from build123d import *

# Parameters (mm, degrees)
F0_W        = 9.525
F0_H        = 112.7125
F1_DEPTH    = 1.5875
F2_T1_DEPTH = 26.9875
F4_D        = 3.175


# Not quite as in the source:
# - a fillet or chamfer that OpenCascade refuses, or shapes differently, is made with other operations: its cross-section is extruded or revolved along the edge and cut away or added


with BuildPart() as f1:
    # F0 (on Top) → F1 (new body)
    with BuildSketch(Plane.XY):
        with Locations((0, 56.35625)):
            Rectangle(F0_W, F0_H)
    extrude(amount=F1_DEPTH)

    # F2: fillet of radius 5.08 on 4 edges, made by hand

    # F2_s2 → F2_t1 (cut)
    with BuildSketch(Plane.XY.offset(-12.7)):
        with BuildLine():
            ThreePointArc((-0.3175, 0), (3.2746024484, 1.4878975516), (4.7625, 5.08))
            Line((4.7625, 5.08), (4.7625, 0))
            Line((4.7625, 0), (-0.3175, 0))
        make_face()
        with BuildLine():
            ThreePointArc((-4.7625, 5.08), (-3.2746024484, 1.4878975516), (0.3175, 0))
            Line((0.3175, 0), (-4.7625, 0))
            Line((-4.7625, 0), (-4.7625, 5.08))
        make_face()
        with BuildLine():
            ThreePointArc((-0.3175, 112.7125), (3.2746024484, 111.2246024484), (4.7625, 107.6325))
            Line((4.7625, 107.6325), (4.7625, 112.7125))
            Line((4.7625, 112.7125), (-0.3175, 112.7125))
        make_face()
        with BuildLine():
            ThreePointArc((0.3175, 112.7125), (-3.2746024484, 111.2246024484), (-4.7625, 107.6325))
            Line((-4.7625, 107.6325), (-4.7625, 112.7125))
            Line((-4.7625, 112.7125), (0.3175, 112.7125))
        make_face()
    extrude(amount=F2_T1_DEPTH, mode=Mode.SUBTRACT)

    # F4 (through all)
    with Locations(Plane.XY.offset(1.5875)):
        with Locations((0, 5.08)):
            Hole(F4_D / 2)


solid = f1.part
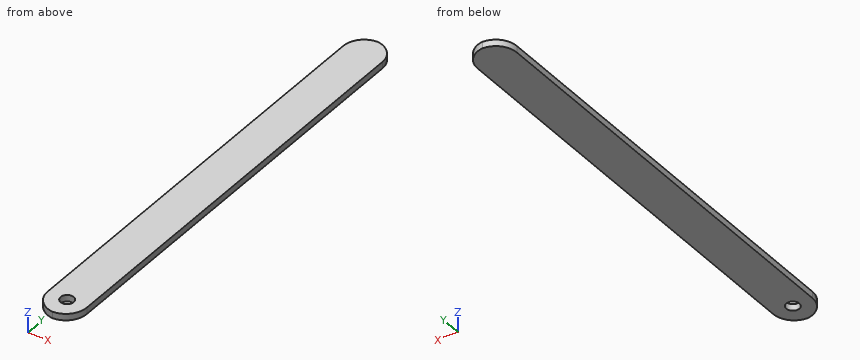
Design review of the part built by this model. Coordinates are the model's own, in mm. Coordinates: 2 decimals unless noted, no trailing zeros. Write each loop counter-clockwise with the first axis right and the second up, starting at its lowest first coordinate (ties: lowest second). Pieces come first, ordered by that corner, then holes. Notation, with made-up numbers: (-0.75, 10.25) - (35.25, 10.25) arc R10 ccw to (35.25, 18.25) - close; hole circle Ø11 at (15.25, -25). An arc over 180 degrees is marked (long way). Use one line per item in the form item = value.
Q1. Consider section A-A (z = 1.1). Write out the cut boundary in (x, y) (1 decimal), plus the area to 3 significant figures.
Taken from the geometry:
outline = (-4.8, 5.1) arc R5.1 ccw to (0, 0) arc R5.1 ccw to (4.8, 5.1) - (4.8, 107.6) arc R5.1 ccw to (0, 112.7) arc R5.1 ccw to (-4.8, 107.6) - close; hole circle Ø3.2 at (0, 5.1)
area = 1,040 mm^2
Q2. Consider section B-B (x = -3.25). Write out the cut boundary in (y, z).
Taken from the geometry:
outline = (1.46, 0) - (111.25, 0) - (111.25, 1.59) - (1.46, 1.59) - close
Q3. Insertion check: pin 1 Ø2.5 at (x, y) = (0, 5.08) entering from -Z. The pin has a flat end and moves straight along its axis. Give the tip position at first contact, or say it passes through.
Taken from the geometry:
pin_1 = through
Q4. For probe 1 along Y at (x, z) = (0.25, 0.8); probe 2 along Y at (x, z) = (-1, 0.3); probe 3 along Y at (x, z) = (-4, 0.55), list the stretches that pass through material, from the lowest coordinate up.
Taken from the geometry:
probe_1 = 0.03 to 3.51, 6.65 to 112.68
probe_2 = 0.17 to 3.85, 6.31 to 112.54
probe_3 = 2.4 to 110.31
